```python
from build123d import *

# Parameters (mm, degrees)
SKETCH1_W           = 46
SKETCH1_H           = 46
SKETCH1_R           = 1
BOSS_EXTRUDE1_DEPTH = 20
FILLET1_R           = 2


with BuildPart() as part:
    # Sketch1 → Boss-Extrude1 (new body)
    with BuildSketch(Plane(origin=(0, 0, 0), x_dir=(1, 0, 0), z_dir=(0, 1, 0))):
        Rectangle(SKETCH1_W, SKETCH1_H)
        with Locations((-20, 20)):
            Circle(SKETCH1_R, mode=Mode.SUBTRACT)
        with Locations((20, 20)):
            Circle(SKETCH1_R, mode=Mode.SUBTRACT)
        with Locations((20, -20)):
            Circle(SKETCH1_R, mode=Mode.SUBTRACT)
        with Locations((-20, -20)):
            Circle(SKETCH1_R, mode=Mode.SUBTRACT)
        with BuildLine():
            Line((-18.881966011, 21), (18.881966011, 21))
            ThreePointArc((18.881966011, 21), (18.939339828, 18.939339828), (21, 18.881966011))
            Line((21, 18.881966011), (21, -18.881966011))
            ThreePointArc((21, -18.881966011), (18.939339828, -18.939339828), (18.881966011, -21))
            Line((18.881966011, -21), (-18.881966011, -21))
            ThreePointArc((-18.881966011, -21), (-18.939339828, -18.939339828), (-21, -18.881966011))
            Line((-21, -18.881966011), (-21, 18.881966011))
            ThreePointArc((-21, 18.881966011), (-18.939339828, 18.939339828), (-18.881966011, 21))
        make_face(mode=Mode.SUBTRACT)
    extrude(amount=BOSS_EXTRUDE1_DEPTH)

    # Fillet1
    fillet1_edges = [part.edges().sort_by_distance(p)[0] for p in [
        (23, 10, 23),
        (-23, 10, 23),
        (-23, 10, -23),
        (23, 10, -23),
    ]]
    fillet(fillet1_edges, radius=FILLET1_R)


solid = part.part
```
The model under review builds one solid part; all positions refer to its coordinate system, in mm. A direction names the side the tool comes from. Give positions to 0.01 mm unless a question says otherwise; leave off trailing zeros. Write each loop counter-clockwise with the first axis right and the second up, starting at its lowest first coordinate (ties: lowest second). Pieces come first, ordered by that corner, then holes. Notation, with made-up numbers: (14.25, 37) - (68.25, 37) arc R15 cw to (68.25, 42) - close; hole circle Ø2 at (37.25, -17). An arc over 180 degrees is marked (long way). Answer in a Markdown table with one row per item. Add a question column.
1. We need section C-C on y = 1.5. Write out the cut boundary in (x, z).
2. We need section A-A on x = -20. Write out the cut boundary in (y, z), then the cut area to 3 significant figures.
3. Tool access review of faces 5 (the flat face through (0, 10, -23)), 6 (the flat face through (0, 10, 21)): name each direction out of +Z, -Z, +X, -X, +Y, -Y from which nothing blocks a thin tool from reaching the whole face with its end or side.
4. Draft analysis for pull direction Z (two halves, no side actions). For faces 1 (the flat face through (21, 10, 0)), 2 (the cylindrical face through (-22.43, 10.14, -22.4)), 3 (the cylindrical face through (-22.43, 10.14, 22.4)), 4 (the flat face through (-2, 20, 22)), state which applies: +Z half, -Z half, draft (parallel to the pull), parting line (faces both ways), or undercut.
5. We need section B-B on z = -20. Write out the cut boundary in (x, y).
6. Insertion check: P1, Ø1.6, axis at x = -20, z = -20, coming from the +Y side. The pin has a flat end and moves straight along its axis. Give the tip position at first contact, or say it passes through.
7. We need section D-D on z = 13. Write out the cut boundary in (x, y).
8. Wall thickness on line 1 along Z through (x, y) = (20, 11.5); line 2 along Z through (x, y) = (-12, 4.5): over which ranges is each line inside the solid? List them lowest first. Write a range as [from, to].
Ans:
| question | item | result |
|---|---|---|
| 1 | outline | (-23, -21) arc R2 ccw to (-21, -23) - (21, -23) arc R2 ccw to (23, -21) - (23, 21) arc R2 ccw to (21, 23) - (-21, 23) arc R2 ccw to (-23, 21) - close; hole circle Ø2 at (-20, -20); hole (-21, -18.88) arc R1.5 cw to (-18.88, -21) - (18.88, -21) arc R1.5 cw to (21, -18.88) - (21, 18.88) arc R1.5 cw to (18.88, 21) - (-18.88, 21) arc R1.5 cw to (-21, 18.88) - close; hole circle Ø2 at (-20, 20); hole circle Ø2 at (20, -20); hole circle Ø2 at (20, 20) |
| 2 | outline | (0, -23) - (20, -23) - (20, -21) - (0, -21) - close; (0, -19) - (20, -19) - (20, -18.5) - (0, -18.5) - close; (0, 18.5) - (20, 18.5) - (20, 19) - (0, 19) - close; (0, 21) - (20, 21) - (20, 23) - (0, 23) - close |
| 2 | area | 100 mm^2 |
| 3 | face 5 | -Z, +X, -X, +Y, -Y |
| 3 | face 6 | +Y, -Y |
| 4 | face 1 | undercut |
| 4 | face 2 | -Z half |
| 4 | face 3 | +Z half |
| 4 | face 4 | draft |
| 5 | outline | (-23, 0) - (-21, 0) - (-21, 20) - (-23, 20) - close; (-19, 0) - (-18.5, 0) - (-18.5, 20) - (-19, 20) - close; (18.5, 0) - (19, 0) - (19, 20) - (18.5, 20) - close; (21, 0) - (23, 0) - (23, 20) - (21, 20) - close |
| 6 | P1 | passes through |
| 7 | outline | (-23, 0) - (-21, 0) - (-21, 20) - (-23, 20) - close; (21, 0) - (23, 0) - (23, 20) - (21, 20) - close |
| 8 | line 1 | z = [-23, -21], [-19, -18.5], [18.5, 19], [21, 23] |
| 8 | line 2 | z = [-23, -21], [21, 23] |
